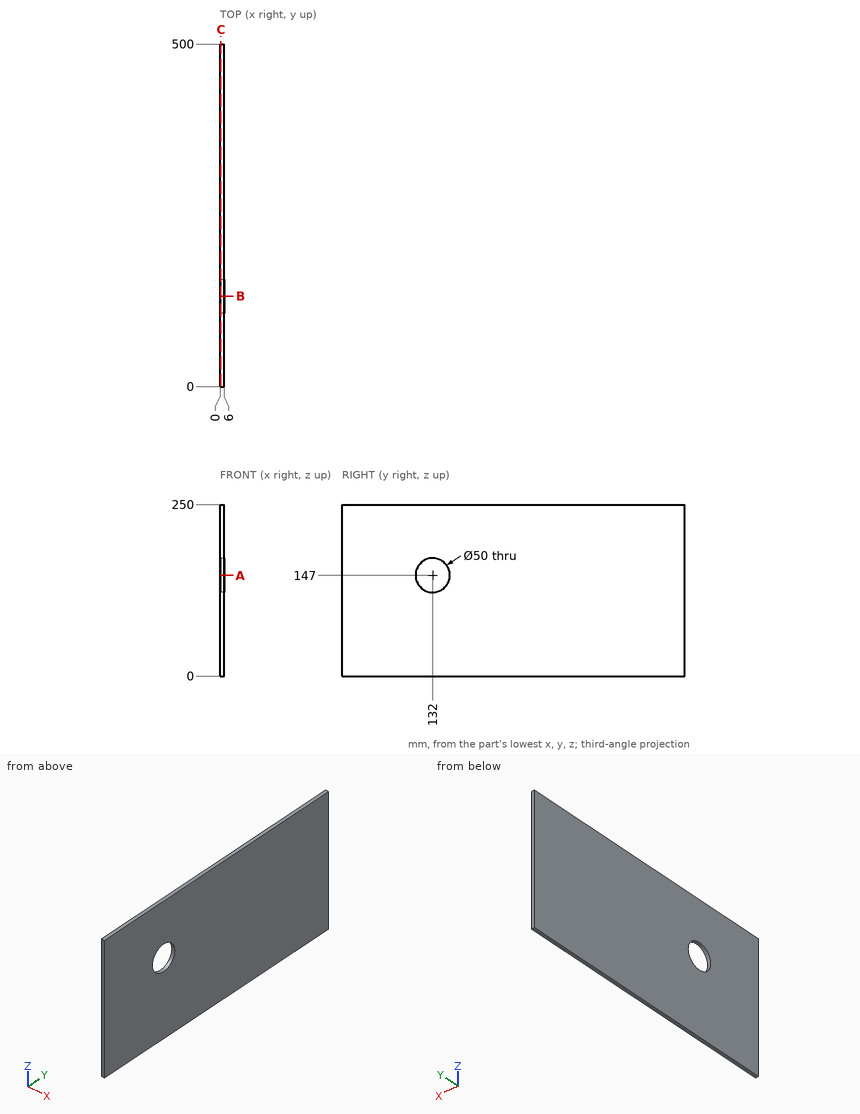
Design review of the part shown in the three views and the two pictorial views. Dimensions are in mm from the part's minimum x, y and z. Round coordinates to 2 decimals unless told otherwise and drop trailing zeros. Loops run counter-clockwise (first coordinate to the right, second up) from the corner with the lowest first, then second, coordinate; pieces in that order, holes last. Notation, with made-up numbers: (-21, -35.75) - (-11, -35.75) arc R18 ccw to (-11, -9.75) - close; hole circle Ø11 at (81, 74.25). An arc over 180 degrees is marked (long way). One line per item, written item: value. Start each with the question number.
Item 1: Take a section at C-C (x = 1.05). Give the boundary of the cut face in (y, z).
Item 2: For L1, parallel to Z at x = 3.4, y = 132; L2, parallel to Z at x = 5.2, y = 116.5; L3, parallel to Y at x = 1.4, z = 161, list the stretches that pass through material, from the lowest coordinate up.
Item 3: Clearance check with a flat-ended pin moving along its axis: pin 1 Ø1.5 at (x, y) = (1.5, 184) entering from -Z. State where the tip first meets the part, or that it passes through.
Item 4: Take a section at A-A (z = 147). Give the boundary of the cut face in (x, y), plus the area to 3 significant figures.
Item 5: Take a section at B-B (y = 132). Give the boundary of the cut face in (x, z), plus the area to 3 significant figures.
Answer below:
1. outline: (0, 0) - (500, 0) - (500, 250) - (0, 250) - close; hole circle Ø50 at (132, 147)
2. L1: z = 0 to 122, 172 to 250
2. L2: z = 0 to 127.38, 166.62 to 250
2. L3: y = 0 to 111.29, 152.71 to 500
3. pin 1: stops at z = 0
4. outline: (0, 0) - (6, 0) - (6, 107) - (0, 107) - close; (0, 157) - (6, 157) - (6, 500) - (0, 500) - close
4. area: 2,700 mm2
5. outline: (0, 0) - (6, 0) - (6, 122) - (0, 122) - close; (0, 172) - (6, 172) - (6, 250) - (0, 250) - close
5. area: 1,200 mm2
